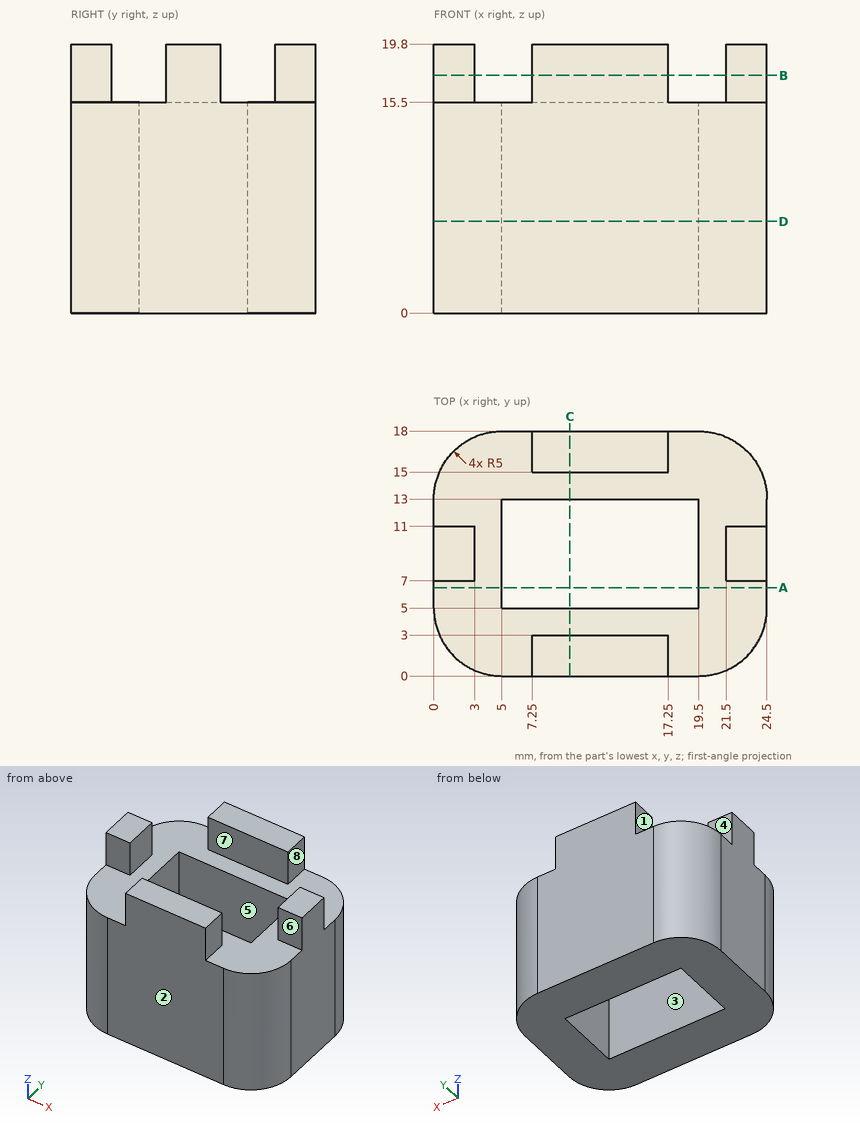
For this review, use the dimensioned drawing (mm, ordinates from the lowest corner) and the shaded views. A direction names the side the tool comes from. Coordinates: 2 decimals unless noted, no trailing zeros. Order: outer loops, then holes, each group sorted by start corner. A loop starts at its lowest first (then second) coordinate and runs counter-clockwise, first axis right, second up. Notation, with made-up numbers: (2, -21.5) - (7, -21.5) arc R13 ccw to (7, 1.5) - close; hole circle Ø10 at (-26, -25). An arc over 180 degrees is marked (long way). Answer as a JSON object with one key per item and string values. Group by question number.
1. Clearance check with flat-ended pins moving along their axes: P1, Ø1.5, axis at y = 14.5, z = 11, coming from the -X side; P2, Ø0.9, axis at y = 17, z = 18, coming from the +X side; P3, Ø3.5, axis at y = 1.5, z = 17.5, coming from the -X side. State where each tip first meets the part, or that it passes through.
2. For probe 1 along X at (y, z) = (7.75, 8.25); probe 2 along Y at (x, z) = (11.5, 12.5); probe 3 along Y at (x, z) = (14.75, 18), list the stretches that pass through material, from the lowest coordinate up.
3. We need section A-A on y = 6.5. State the section outline as (x, z) points, then the cut area to 3 significant figures.
4. For the marked faces 5, 6, 7 and 8, list the 3-axis set-ups (+Z, -Z, +X, -X, +Y, -Y) from which the entire face can be reached by the end or side of a thin tool; tool diameter is ignored.
5. We need section D-D on z = 6.75. State the section outline as (x, y) points, then the cut area to 3 significant figures.
6. The part is to be moulded in two halves that separate along Y. For the marked faces 1, 2, 3 and 4, say which applies: pulls with the +Y half, pulls with the -Y half, needs draft (parallel to the pull), parting line crosses it, or undercut.
7. We need section B-B on z = 17.5. State the section outline as (x, y) points, then the cut area to 3 significant figures.
8. We need section C-C on x = 10. State the section outline as (y, z) points, then the cut area to 3 significant figures.
Final values:
{
 "1": {"P1": "x = 0.06", "P2": "x = 17.25", "P3": "x = 7.25"},
 "2": {"probe 1": "0 to 5, 19.5 to 24.5", "probe 2": "0 to 5, 13 to 18", "probe 3": "0 to 3, 15 to 18"},
 "3": {"outline": "(0, 0) - (5, 0) - (5, 15.5) - (0, 15.5) - close; (19.5, 0) - (24.5, 0) - (24.5, 15.5) - (19.5, 15.5) - close", "area": "155 mm²"},
 "4": {"face 5": "+Z, -Z", "face 6": "+Z, +X, -X, -Y", "face 7": "+Z, +X, -X", "face 8": "+Z, +X, +Y, -Y"},
 "5": {"outline": "(0, 5) arc R5 ccw to (5, 0) - (19.5, 0) arc R5 ccw to (24.5, 5) - (24.5, 13) arc R5 ccw to (19.5, 18) - (5, 18) arc R5 ccw to (0, 13) - close; hole (5, 5) - (19.5, 5) - (19.5, 13) - (5, 13) - close", "area": "304 mm²"},
 "6": {"face 1": "needs draft", "face 2": "pulls with the -Y half", "face 3": "undercut", "face 4": "pulls with the +Y half"},
 "7": {"outline": "(0, 7) - (3, 7) - (3, 11) - (0, 11) - close; (7.25, 0) - (17.25, 0) - (17.25, 3) - (7.25, 3) - close; (7.25, 15) - (17.25, 15) - (17.25, 18) - (7.25, 18) - close; (21.5, 7) - (24.5, 7) - (24.5, 11) - (21.5, 11) - close", "area": "84.0 mm²"},
 "8": {"outline": "(0, 0) - (5, 0) - (5, 15.5) - (3, 15.5) - (3, 19.8) - (0, 19.8) - close; (13, 0) - (18, 0) - (18, 19.8) - (15, 19.8) - (15, 15.5) - (13, 15.5) - close", "area": "181 mm²"}
}
